from build123d import *

# Parameters (mm, degrees)
SKETCH2_R                                       = 50
BOSS_EXTRUDE1_DEPTH                             = 12
CSK_FOR_M5_FLAT_HEAD_MACHINE_SCREW1_D           = 5.5
CSK_FOR_M5_FLAT_HEAD_MACHINE_SCREW1_DEPTH       = 12
CSK_FOR_M5_FLAT_HEAD_MACHINE_SCREW1_CSINK_D     = 10.4
CSK_FOR_M5_FLAT_HEAD_MACHINE_SCREW1_CSINK_ANGLE = 90
SKETCH6_R                                       = 3
CUT_EXTRUDE1_DEPTH                              = 1
CHAMFER1_SIZE                                   = 2


with BuildPart() as part:
    # Sketch2 → Boss-Extrude1 (new body)
    with BuildSketch(Plane.XY):
        Circle(SKETCH2_R)
    extrude(amount=BOSS_EXTRUDE1_DEPTH)

    # CSK for M5 Flat Head Machine Screw1
    with Locations(Plane.XY.offset(12)):
        with Locations((0, 35)):
            CounterSinkHole(CSK_FOR_M5_FLAT_HEAD_MACHINE_SCREW1_D / 2, CSK_FOR_M5_FLAT_HEAD_MACHINE_SCREW1_CSINK_D / 2, depth=CSK_FOR_M5_FLAT_HEAD_MACHINE_SCREW1_DEPTH, counter_sink_angle=CSK_FOR_M5_FLAT_HEAD_MACHINE_SCREW1_CSINK_ANGLE)

    # Sketch6 → Cut-Extrude1 (cut)
    with BuildSketch(Plane.XY.offset(12)):
        with Locations((-28.425692604, 28.425692604)):
            Circle(SKETCH6_R)
        with Locations((28.425692604, 28.425692604)):
            Circle(SKETCH6_R)
        with Locations((28.425692604, -28.425692604)):
            Circle(SKETCH6_R)
        with Locations((-28.425692604, -28.425692604)):
            Circle(SKETCH6_R)
    extrude(amount=-CUT_EXTRUDE1_DEPTH, mode=Mode.SUBTRACT)

    # Chamfer1
    chamfer1_edges = [part.edges().sort_by_distance(p)[0] for p in [
        (-50, 0, 12),
    ]]
    chamfer(chamfer1_edges, length=CHAMFER1_SIZE)


solid = part.part
Check sheet for the modelled part. Datum: model origin and axes. Units: mm. A direction names the side the tool comes from. Give positions to 0.01 mm unless a question says otherwise; leave off trailing zeros. Order: outer loops, then holes, each group sorted by start corner. A loop starts at its lowest first (then second) coordinate and runs counter-clockwise, first axis right, second up. Notation, with made-up numbers: M 17.25,81.5 L 23.25,81.5 A23 cw 23.25,96.5 Z; hole C 26.25,-34 d8. An arc over 180 degrees is marked long. Answer as CSV lines item,"result". Start each with the question number.
Item 1: Thickness scan on line 1 (Y direction, x = 0, z = 7.75); line 2 (Z direction, x = -29, y = -27); line 3 (Y direction, x = -1.5, z = 1.75). Record the ranges inside material, lowest first. Write a range as [from, to].
Item 2: Cross-section at A-A on x = 0. Enter the section's corners in (y, z).
Item 3: Gauge pin test, flat ends, axial feed: P1, Ø5.5, axis at x = 28.43, y = -28.43, coming from the -Z side; P2, Ø4, axis at x = 22, z = 10, coming from the +Y side; P3, Ø1.8, axis at x = -28, y = 29, coming from the +Z side; P4, Ø9, axis at x = 0, y = 35, coming from the +Z side. Record the tip position at first contact, or that the pin passes through.
Item 4: Mould release check, pull along Y, two halves, no side actions. Record for faces 1 (the face through (-28, 28, 11)), 2 (the face through (28, -28, 11)), 3 (the face through (-1, 1, 0)), 4 (the face through (47.69, 15.02, 4.93)): +Y half, -Y half, draft (parallel to the pull), parting line (faces both ways), or undercut.
Item 5: Tool access check on faces 5 (the face through (-28.82, 31.4, 11.51)), 6 (the face through (0.358, 37.727, 4.708)). Record the directions out of +Z, -Z, +X, -X, +Y, -Y that give a thin tool (end or side, any length) a straight path to the whole face; none if there is none.
Item 6: Cross-section at B-B on z = 4.5. Enter the section's corners in (x, y).
Established:
1,line 1,"y = [-50, 32.25], [37.75, 50]"
1,line 2,"z = [0, 11]"
1,line 3,"y = [-49.98, 32.7], [37.3, 49.98]"
2,outline,"M -50,0 L 32.25,0 L 32.25,9.55 L 29.8,12 L -48,12 L -50,10 Z; M 37.75,0 L 50,0 L 50,10 L 48,12 L 40.2,12 L 37.75,9.55 Z"
3,P1,"stops at z = 0"
3,P2,"stops at y = 45.83"
3,P3,"stops at z = 11"
3,P4,"stops at z = 11.3"
4,face 1,"undercut"
4,face 2,"undercut"
4,face 3,"draft"
4,face 4,"parting line"
5,face 5,"+Z"
5,face 6,"+Z, -Z"
6,outline,"C 0,0 d100; hole C 0,35 d5.5"
